For this review, use the dimensioned drawing (mm, ordinates from the lowest corner) and the shaded views. Round coordinates to 2 decimals unless told otherwise and drop trailing zeros. Write each loop counter-clockwise with the first axis right and the second up, starting at its lowest first coordinate (ties: lowest second). Pieces come first, ordered by that corner, then holes.
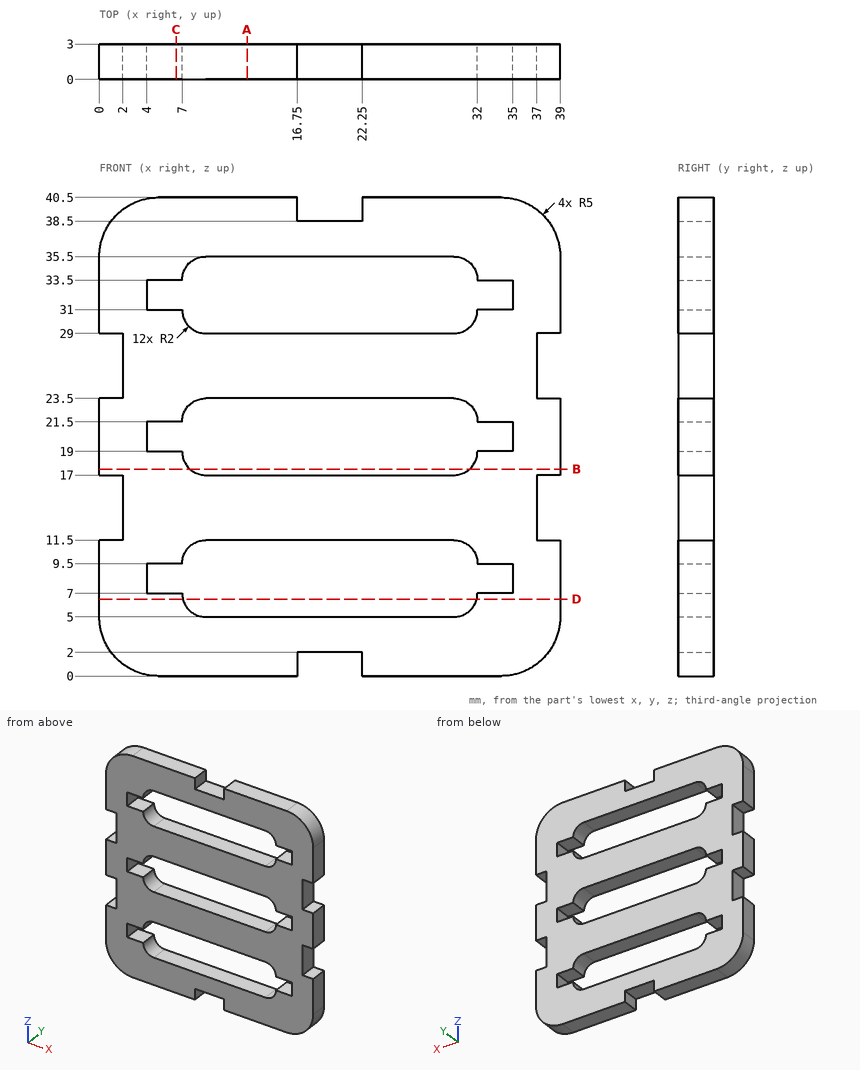
(1) We need section A-A, the plane x = 12.5. Give the boundary of the cut face in (y, z).
Geometry check:
outline: (0, 0) - (3, 0) - (3, 5) - (0, 5) - close; (0, 11.5) - (3, 11.5) - (3, 17) - (0, 17) - close; (0, 23.5) - (3, 23.5) - (3, 29) - (0, 29) - close; (0, 35.5) - (3, 35.5) - (3, 40.5) - (0, 40.5) - close
(2) We need section C-C, the plane x = 6.5. Give the boundary of the cut face in (y, z).
Geometry check:
outline: (0, 0) - (3, 0) - (3, 7) - (0, 7) - close; (0, 9.5) - (3, 9.5) - (3, 19) - (0, 19) - close; (0, 21.5) - (3, 21.5) - (3, 31) - (0, 31) - close; (0, 33.5) - (3, 33.5) - (3, 40.5) - (0, 40.5) - close
(3) We need section D-D, the plane z = 6.5. Give the boundary of the cut face in (x, y).
Geometry check:
outline: (0, 0) - (7.06, 0) - (7.06, 3) - (0, 3) - close; (31.94, 0) - (39, 0) - (39, 3) - (31.94, 3) - close
(4) We need section B-B, the plane z = 17.5. Give the boundary of the cut face in (x, y).
Geometry check:
outline: (0, 0) - (7.68, 0) - (7.68, 3) - (0, 3) - close; (31.32, 0) - (39, 0) - (39, 3) - (31.32, 3) - close
(5) For line 1 along Z through (x, y) = (16.5, 2.4); line 2 along Z through (x, y) = (5.5, 2.35); line 3 along X through (y, z) = (2.9, 19.5), list the stretches that pass through material, from the lowest coordinate up.
Geometry check:
line 1: z = 0 to 5, 11.5 to 17, 23.5 to 29, 35.5 to 40.5
line 2: z = 0 to 7, 9.5 to 19, 21.5 to 31, 33.5 to 40.5
line 3: x = 0 to 4, 35 to 39
(6) For pin 1 Ø1 at (x, y) = (1.5, 1) entering from -Z; pin 2 Ø1 at (x, y) = (38, 1.5) entering from -Z, all flat-tipped, find the tip position at first contact; note any pin that passes through.
Geometry check:
pin 1: stops at z = 1
pin 2: stops at z = 1.43
